```python
from build123d import *

# Parameters (mm, degrees)
F0_R     = 4
F1_DEPTH = 18
F0_W     = 18
F0_H     = 100
F2_DEPTH = 9


with BuildPart() as f1:
    # F0 (on Front) → F1 (new body)
    with BuildSketch(Plane.XZ):
        with BuildLine():
            Line((-59.240983, 23.115967), (-59.240983, 115.115967))
            ThreePointArc((-59.240983, 115.115967), (-60.412556, 117.944394), (-63.240983, 119.115967))
            Line((-63.240983, 119.115967), (-91.240983, 119.115967))
            Line((-91.240983, 119.115967), (-91.240983, 19.115967))
            Line((-91.240983, 19.115967), (-63.240983, 19.115967))
            ThreePointArc((-63.240983, 19.115967), (-60.412556, 20.287539), (-59.240983, 23.115967))
        make_face()
        with Locations((-74.740983, 34.115967)):
            Circle(F0_R, mode=Mode.SUBTRACT)
        with Locations((-74.740983, 104.115967)):
            Circle(F0_R, mode=Mode.SUBTRACT)
    extrude(amount=F1_DEPTH)

    # F0 (on Front) → F2 (join)
    with BuildSketch(Plane.XZ):
        with Locations((-100.240983, 69.115967)):
            Rectangle(F0_W, F0_H)
    extrude(amount=F2_DEPTH)


solid = f1.part
```
Here's how the part is built. I have some questions about the finished solid (model axes, mm). A direction names the side the tool comes from. Give positions to 0.01 mm unless a question says otherwise; leave off trailing zeros. Write each loop counter-clockwise with the first axis right and the second up, starting at its lowest first coordinate (ties: lowest second). Pieces come first, ordered by that corner, then holes. Notation, with made-up numbers: (-6, -34.5) -> (11, -34.5) arc R12 cw to (11, -17.5) -> close; hole circle Ø6 at (-12, -36). An arc over 180 degrees is marked (long way). Write each question's results on one line, items separated by ' | '.
Item 1: Suppose I cut it at B-B on z = 82.5. Write out the boundary of the cut face in (x, y).
Output:
outline: (-109.24, -9) -> (-91.24, -9) -> (-91.24, -18) -> (-59.24, -18) -> (-59.24, 0) -> (-109.24, 0) -> close
Item 2: On a 3-axis mill with a long thin cutter (end or side, diameter ignored), from which of +Z, -Z, +X, -X, +Y, -Y can I reach the whole of each face in a straight line? I mean faces 5 (the face through (-100, -9, 70)), 6 (the face through (-81, -7, 119.116)). Say none if no direction works.
Output:
face 5: +Z, -Z, -X, -Y | face 6: +Z, +X, -X, +Y, -Y
Item 3: Suppose I cut it at C-C on y = -15.75. Write out the boundary of the cut face in (x, z), plus the area to 3 significant figures.
Output:
outline: (-91.24, 19.12) -> (-63.24, 19.12) arc R4 ccw to (-59.24, 23.12) -> (-59.24, 115.12) arc R4 ccw to (-63.24, 119.12) -> (-91.24, 119.12) -> close; hole circle Ø8 at (-74.74, 34.12); hole circle Ø8 at (-74.74, 104.12) | area: 3,090 mm^2
Item 4: If I drill on L1, parallel to Z at x = -71.5, y = -8.5; L2, parallel to Y at x = -106, z = 66.5; L3, parallel to X at y = -13.25, z = 59.5, over which ranges is the centre line in solid material (lowest first)?
Output:
L1: z = 19.12 to 31.77, 36.46 to 101.77, 106.46 to 119.12 | L2: y = -9 to 0 | L3: x = -91.24 to -59.24
Item 5: Suppose I cut it at A-A on z = 106. Write out the boundary of the cut face in (x, y).
Output:
outline: (-109.24, -9) -> (-91.24, -9) -> (-91.24, -18) -> (-78.27, -18) -> (-78.27, 0) -> (-109.24, 0) -> close; (-71.21, -18) -> (-59.24, -18) -> (-59.24, 0) -> (-71.21, 0) -> close
Item 6: Suppose I cut it at D-D on x = -96.5. Write out the boundary of the cut face in (y, z), plus the area to 3 significant figures.
Output:
outline: (-9, 19.12) -> (0, 19.12) -> (0, 119.12) -> (-9, 119.12) -> close | area: 900 mm^2
Item 7: We'd pull the mould along X, two halves only. Please class faces 1 (the face through (-77.69, -8.87, 36.82)), 2 (the face through (-77.69, -8.87, 106.82)), 3 (the face through (-91.241, -13, 70)), 4 (the face through (-81, -7, 19.116)): pulls with the +X half, pulls with the -X half, needs draft (parallel to the pull), parting line crosses it, or undercut.
Output:
face 1: undercut | face 2: undercut | face 3: pulls with the -X half | face 4: needs draft
Item 8: For pin 1 Ø20 at (x, z) = (-104, 63.5) entering from -Y; pin 2 Ø2.5 at (y, z) = (-12.5, 84) entering from -X, each with a flat end and sliding along its axis, tell me the tip position at first contact or that it passes through.
Output:
pin 1: stops at y = -9 | pin 2: stops at x = -91.24
